Could you check a few things on this model? Use its own coordinates, in mm. A direction names the side the tool comes from. Round coordinates to 2 decimals unless told otherwise and drop trailing zeros. Write each loop counter-clockwise with the first axis right and the second up, starting at its lowest first coordinate (ties: lowest second). Pieces come first, ordered by that corner, then holes.
```python
from build123d import *

# Parameters (mm, degrees)
SKETCH5_R           = 30.1117
BOSS_EXTRUDE3_DEPTH = 2.54
BOSS_EXTRUDE4_DEPTH = 1.905
CIRPATTERN2_COUNT   = 6
SKETCH8_R           = 34.925
SKETCH8_R_2         = 30.1117
SKETCH8_R_3         = 7.9375
SKETCH8_R_4         = 3.2639
CUT_EXTRUDE3_DEPTH  = 46.107338309
SKETCH9_R           = 7.9375
SKETCH9_R_2         = 3.2639
BOSS_EXTRUDE5_DEPTH = 2.54


with BuildPart() as part:
    # Sketch5 → Boss-Extrude3 (new body)
    with BuildSketch(Plane(origin=(0, 0, 0), x_dir=(1, 0, 0), z_dir=(0, 1, 0))):
        with Locations(Location((0, 0, 0), (0, 0, 270))):
            Circle(SKETCH5_R)
    extrude(amount=-BOSS_EXTRUDE3_DEPTH)

    # Sketch7 → Boss-Extrude4 (add, symmetric)
    with BuildSketch(Plane.XY):
        Polygon((30.1117, 0), (30.1117, 7.62), (6.35, 12.33424), (6.35, 0), align=None)
    boss_extrude4 = extrude(amount=BOSS_EXTRUDE4_DEPTH, both=True)

    # CirPattern2: Boss-Extrude4 ×6 about axis
    cirpattern2_axis = Axis((0, 0, 0), (0, 1, 0))
    for i in range(1, CIRPATTERN2_COUNT):
        add(boss_extrude4.rotate(cirpattern2_axis, i * 360 / CIRPATTERN2_COUNT))

    # Sketch8 → Cut-Extrude3 (cut, through all)
    # profile 1 of 3: a face of its own
    with BuildSketch(Plane.XZ.offset(2.54)):
        Circle(SKETCH8_R)
        with Locations(Location((0, 0, 0), (0, 0, 90))):
            Circle(SKETCH8_R_2, mode=Mode.SUBTRACT)
    # profile 2 of 3: a face of its own
    with BuildSketch(Plane.XZ.offset(2.54)):
        with Locations(Location((0, 0, 0), (0, 0, 270))):
            Circle(SKETCH8_R_3)
        Circle(SKETCH8_R_4, mode=Mode.SUBTRACT)
    # profile 3 of 3: a face of its own
    with BuildSketch(Plane.XZ.offset(2.54)):
        Circle(SKETCH8_R_4)
    extrude(amount=-CUT_EXTRUDE3_DEPTH, mode=Mode.SUBTRACT)

    # Sketch9 → Boss-Extrude5 (add)
    with BuildSketch(Plane.XZ.offset(2.54)):
        Circle(SKETCH9_R)
        with Locations(Location((0, 0, 0), (0, 0, 270))):
            Circle(SKETCH9_R_2, mode=Mode.SUBTRACT)
    extrude(amount=-BOSS_EXTRUDE5_DEPTH)


solid = part.part
```
Q1. Imagine slicing it at B-B, the plane y = 4. Write out the boundary of the cut face in (x, z) (1 decimal).
Q2. Imagine slicing it at C-C, the plane z = 0. Write out the boundary of the cut face in (x, y).
Q3. Imagine slicing it at D-D, the plane x = -12.5. Write out the boundary of the cut face in (y, z) (3 decimals).
Q4. If I drill on L1, parallel to X at y = -1.7, z = 0; L2, parallel to Z at x = 15, y = 5.25 (3 decimals); L3, parallel to Z at x = -8, y = 3.75 (3 decimals), over which ranges is the centre line in solid material (lowest first)?
Q5. I'm going to push flat-ended pins straight in: pin 1 Ø6 at (x, y) = (-21, 8) entering from -Z (3 decimals); pin 2 Ø3 at (x, y) = (-21, 5.5) entering from +Z (3 decimals); pin 3 Ø6 at (x, y) = (-3, 5.5) entering from +Z. Where does each tip first touch, or does it pass through?
Q6. Imagine slicing it at A-A, the plane x = 0. Write out the boundary of the cut face in (y, z), then the cut area to 3 significant figures.
Q7. On a 3-axis mill with a long thin cutter (end or side, diameter ignored), from which of +Z, -Z, +X, -X, +Y, -Y can I reach the whole of each face in a straight line? I mean faces 5 (the flat face through (7.711, 4.777, -17.166)), 6 (the cylindrical face through (-7.937, 5.948, 0.027)), 7 (the flat face through (7.711, 4.777, 17.166)), 8 (the flat face through (19, 5, -1.905)), 9 (the flat face through (11.01, 4.78, -15.26)). Say none if no direction works.
Q8. We'd pull the mould along X, two halves only. Please class faces 1 (the cylindrical face through (-3.186, -1.288, 0.708)), 2 (the flat face through (-11.01, 4.78, -15.26)), 3 (the cylindrical face through (3.99, 5.95, 6.86)), 4 (the cylindrical face through (-16.176, 0.262, 25.398)): pulls with the +X half, pulls with the -X half, needs draft (parallel to the pull), parting line crosses it, or undercut.
Results found:
1. outline: (-30.1, -1.9) - (-7.7, -1.9) arc R7.9 cw to (-7.7, 1.9) - (-30.1, 1.9) arc R30.1 ccw to start; (-16.7, -25.1) arc R30.1 ccw to (-13.4, -27) - (-2.2, -7.6) arc R7.9 cw to (-5.5, -5.7) - close; (-16.7, 25.1) - (-5.5, 5.7) arc R7.9 cw to (-2.2, 7.6) - (-13.4, 27) arc R30.1 ccw to start; (2.2, -7.6) - (13.4, -27) arc R30.1 ccw to (16.7, -25.1) - (5.5, -5.7) arc R7.9 cw to start; (2.2, 7.6) arc R7.9 cw to (5.5, 5.7) - (16.7, 25.1) arc R30.1 ccw to (13.4, 27) - close; (7.7, -1.9) - (30.1, -1.9) arc R30.1 ccw to (30.1, 1.9) - (7.7, 1.9) arc R7.9 cw to start
2. outline: (-30.11, -2.54) - (-3.26, -2.54) - (-3.26, 0) - (-7.94, 0) - (-7.94, 12.02) - (-30.11, 7.62) - close; (3.26, -2.54) - (30.11, -2.54) - (30.11, 7.62) - (7.94, 12.02) - (7.94, 0) - (3.26, 0) - close
3. outline: (-2.54, -27.395) - (0, -27.395) - (0, -25.461) - (7.98, -25.461) - (9.289, -17.841) - (0, -17.841) - (0, -1.905) - (11.114, -1.905) - (11.114, 1.905) - (0, 1.905) - (0, 17.841) - (9.289, 17.841) - (7.98, 25.461) - (0, 25.461) - (0, 27.395) - (-2.54, 27.395) - close
4. L1: x = -30.11 to -3.26, 3.26 to 30.11
4. L2: z = -26.11 to -22.171, -1.905 to 1.905, 22.171 to 26.11
4. L3: z = -17.666 to -10.046, -1.905 to 1.905, 10.046 to 17.666
5. pin 1: stops at z = -1.905
5. pin 2: stops at z = 1.905
5. pin 3: stops at z = 14.2
6. outline: (-2.54, -30.11) - (0, -30.11) - (0, -3.26) - (-2.54, -3.26) - close; (-2.54, 3.26) - (0, 3.26) - (0, 30.11) - (-2.54, 30.11) - close
6. area: 136 mm2
7. face 5: -Z, +Y
7. face 6: +Y
7. face 7: +Z, +Y
7. face 8: +X, -X, +Y
7. face 9: +X, +Y
8. face 1: undercut
8. face 2: pulls with the -X half
8. face 3: undercut
8. face 4: parting line crosses it
